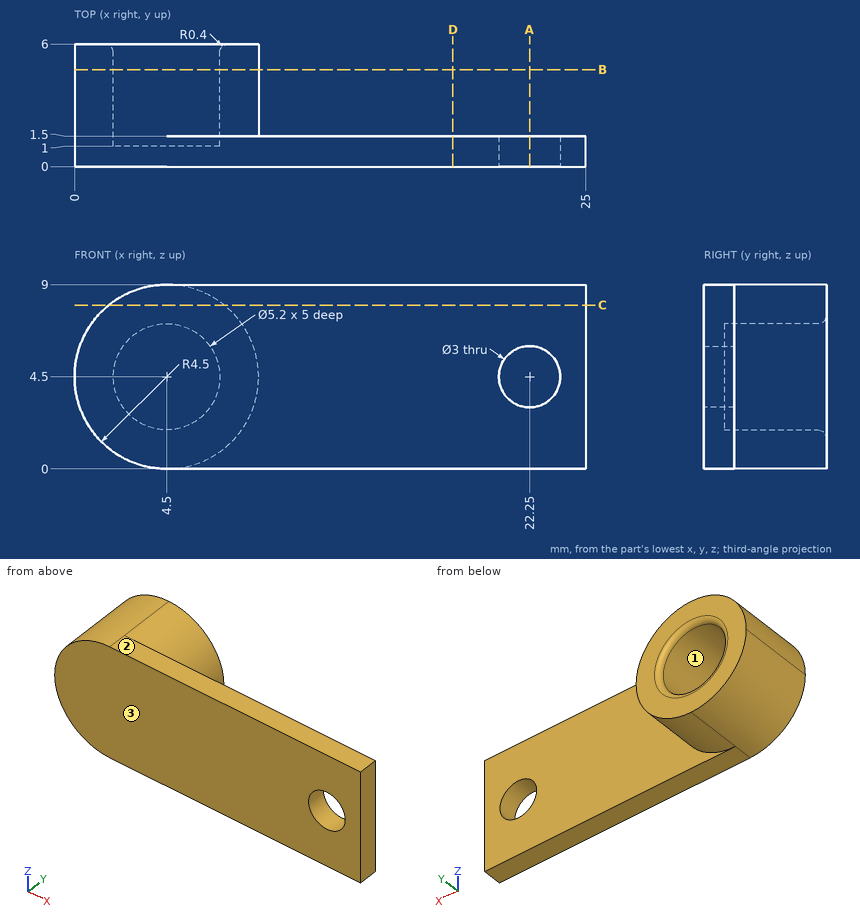
Study the drawing (mm; zero at the part's minimum x, y, z) and answer. Round coordinates to 2 decimals unless told otherwise and drop trailing zeros. Loops run counter-clockwise (first coordinate to the right, second up) from the corner with the lowest first, then second, coordinate; pieces in that order, holes last. Notation, with made-up numbers: (-18.5, 12.5) -> (27.5, 12.5) arc R29 cw to (27.5, 38.5) -> close; hole circle Ø4 at (88.5, 21). An arc over 180 degrees is marked (long way). Write each question's results on one line, items separated by ' | '. Start each with the question number.
1. Section C-C (z = 8) is taken. Determine the outline of the cut face in (x, y).
2. Given pin 1 Ø2.5 at (x, z) = (22.25, 4.5) entering from +Y; pin 2 Ø3 at (x, z) = (4.5, 4.5) entering from +Y; pin 3 Ø2.5 at (x, z) = (16, 3.5) entering from +Y; pin 4 Ø1 at (y, z) = (1, 2.5) entering from -X, each flat-ended and moving along its own axis, determine where each tip first touches the part or whether it passes through.
3. Section B-B (y = 4.75) is taken. Determine the outline of the cut face in (x, z), plus the area to 3 significant figures.
4. Section A-A (x = 22.25) is taken. Determine the outline of the cut face in (y, z), plus the area to 3 significant figures.
5. Section D-D (x = 18.5) is taken. Determine the outline of the cut face in (y, z).
6. For a pull along Z with two mould halves and no side action, classify the marked faces 1, 2 and 3 as +Z half, -Z half, draft (parallel to the pull), parting line (faces both ways), or undercut.
7. Find the intervals of material crossed by probe 1 along Z at (x, y) = (22.25, 1); probe 2 along X at (y, z) = (0.4, 4.5); probe 3 along X at (y, z) = (2.6, 4.5), in increasing order. Write a range as from..to.
Evaluation:
1) outline: (1.67, 0) -> (25, 0) -> (25, 1.5) -> (7.33, 1.5) -> (7.33, 6) -> (1.67, 6) -> close
2) pin 1: passes through | pin 2: stops at y = 1 | pin 3: stops at y = 1.5 | pin 4: stops at x = 0.26
3) outline: circle Ø9 at (4.5, 4.5); hole circle Ø5.2 at (4.5, 4.5) | area: 42.4 mm2
4) outline: (0, 0) -> (1.5, 0) -> (1.5, 3) -> (0, 3) -> close; (0, 6) -> (1.5, 6) -> (1.5, 9) -> (0, 9) -> close | area: 9.00 mm2
5) outline: (0, 0) -> (1.5, 0) -> (1.5, 9) -> (0, 9) -> close
6) face 1: undercut | face 2: +Z half | face 3: draft
7) probe 1: z = 0..3, 6..9 | probe 2: x = 0..20.75, 23.75..25 | probe 3: x = 0..1.9, 7.1..9
